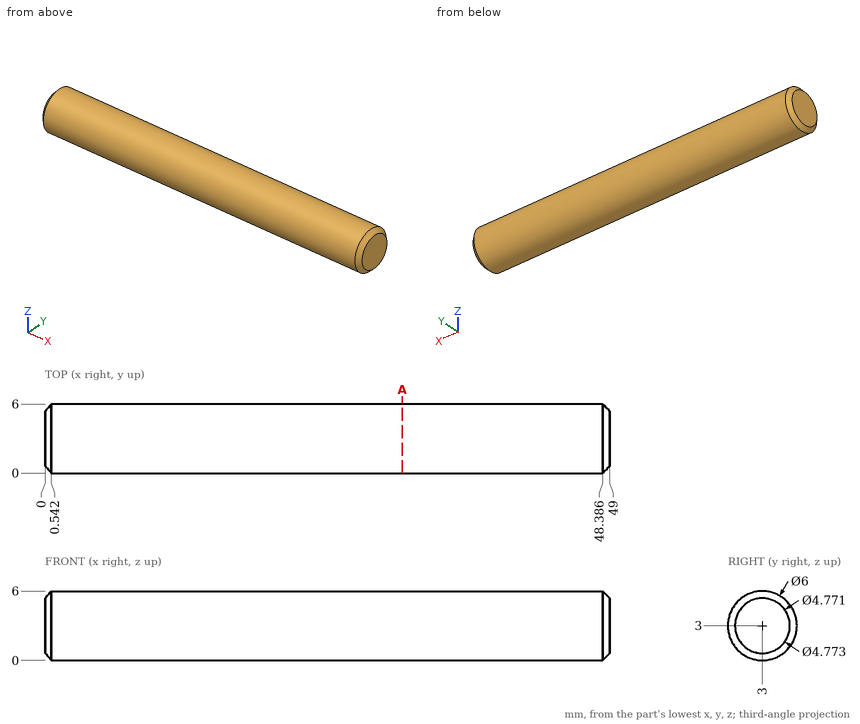
Input: dimensioned drawing with shaded views. Units: mm. Origin: part minimum x, y, z. Give positions to 0.01 mm unless a question says otherwise; leave off trailing zeros. Order: outer loops, then holes, each group sorted by start corner. A loop starts at its lowest first (then second) coordinate and runs counter-clockwise, first axis right, second up.
(1) Section query A-A (x = 31). Return the cut outline in (y, z).
(2) Material intervals for line 1 along Y through (x, z) = (39.5, 2.9); line 2 along Z through (x, y) = (19.5, 4.75) (1 decimal); line 3 along Z through (x, y) = (20.5, 3.25), sorted ascending.
(3) Contact query for a flat-ended pin moving along its axis: P1, Ø3, axis at x = 19, z = 1, coming from the -Y side. Output: stop coordinate, or through.
Outcome:
1. outline: circle Ø6 at (3, 3)
2. line 1: y = 0 to 6
2. line 2: z = 0.6 to 5.4
2. line 3: z = 0.01 to 5.99
3. P1: stops at y = 0.04
